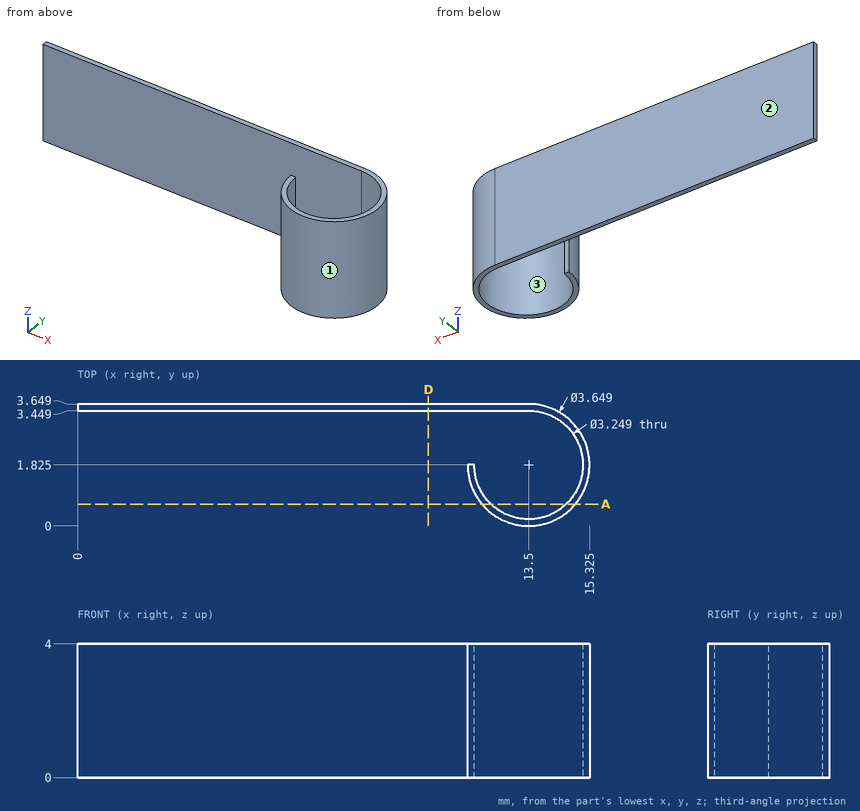
Check sheet for the drawn part. Datum: minimum x, y, z corner. Units: mm. Coordinates: 2 decimals unless noted, no trailing zeros. Loops run counter-clockwise (first coordinate to the right, second up) from the corner with the lowest first, then second, coordinate; pieces in that order, holes last. Notation, with made-up numbers: (-39, 38) -> (-20, 38) arc R33 cw to (-20, 70) -> close; hole circle Ø8 at (32, 55.5). An arc over 180 degrees is marked (long way). Answer as a JSON object with one key per item and string values. Group by question number.
Item 1: Mould release check, pull along Y, two halves, no side actions. Record for the marked faces 1, 2 and 3: +Y half, -Y half, draft (parallel to the pull), parting line (faces both ways), or undercut.
Item 2: Depth check by flat-ended pin: pin 1 (1.5 mm diameter, centred on x = 5.5, y = 1, fed in from -Z); pin 2 (1.5 mm diameter, centred on x = 3.5, y = 3, fed in from +Z). Enter the tip coordinate at first touch or a pass-through.
Item 3: Scan lines: probe 1 along Y at (x, z) = (13.5, 2.45); probe 2 along X at (y, z) = (1.9, 2.85); probe 3 along X at (y, z) = (1.65, 2.8) (1 decimal). Record each from-to range of solid material in increasing order.
Item 4: Sectioned sample at D-D on x = 10.5. Record the boundary of the cut face in (y, z).
Item 5: Sectioned sample at A-A on y = 0.65. Record the boundary of the cut face in (x, z).
Evaluation:
{
 "1": {"face 1": "parting line", "face 2": "+Y half", "face 3": "undercut"},
 "2": {"pin 1": "passes through", "pin 2": "stops at z = 4"},
 "3": {"probe 1": "y = 0 to 0.2, 3.45 to 3.65", "probe 2": "x = 15.12 to 15.32", "probe 3": "x = 11.7 to 11.9, 15.1 to 15.3"},
 "4": {"outline": "(3.45, 0) -> (3.65, 0) -> (3.65, 4) -> (3.45, 4) -> close"},
 "5": {"outline": "(12.1, 0) -> (12.38, 0) -> (12.38, 4) -> (12.1, 4) -> close; (14.62, 0) -> (14.9, 0) -> (14.9, 4) -> (14.62, 4) -> close"}
}
